CAD build for the part. Positions are in the model's coordinates, mm. Face numbers are marked on the shaded views. Coordinates: 2 decimals unless noted, no trailing zeros. Write each loop counter-clockwise with the first axis right and the second up, starting at its lowest first coordinate (ties: lowest second). Pieces come first, ordered by that corner, then holes. Notation, with made-up numbers: (-7.5, 54.5) - (32.5, 54.5) arc R20 ccw to (32.5, 63.5) - close; hole circle Ø8 at (18.5, -22). An arc over 180 degrees is marked (long way). One line per question, with ' | ' between items. Start each with the question number.
1. Two-plate mould, pull along Z, no slides. Class the marked faces 1, 2 and 3: +Z half, -Z half, draft (parallel to the pull), parting line (faces both ways), or undercut.
2. Band-saw the part on D-D, the plane x = -5. Write the cut outline in (y, z) (3 decimals), then the cut area to 3 significant figures.
3. Flat gauge pins, fed straight in: P1, Ø3, axis at x = -3.5, y = 19, coming from the -Z side; P2, Ø5.5, axis at y = 12.7, z = -19.05, coming from the +X side (1 decimal); P3, Ø6, axis at x = 0.5, y = 3, coming from the -Z side; P4, Ø4, axis at x = 4, z = -8, coming from the -Y side. Where does each tip first touch, or does it go through?
4. Band-saw the part on B-B, the plane z = -16.25. Write the cut outline in (x, y), then the cut area to 3 significant figures.
5. Probe line 1 (X direction, y = 8.5, z = -1); line 2 (Z direction, x = 3.75, y = 12.7) (3 decimals); line 3 (Z direction, x = -4.25, y = 23) (3 decimals). List the from-to ranges inside material, lowest first.
6. Band-saw the part on A-A, the plane y = 12.7. Write the cut outline in (x, z) (3 decimals).
7. Band-saw the part on C-C, the plane x = 5. Write the cut outline in (y, z) (3 decimals).
Autodesk Inventor part; units mm, degrees
ref_plane "YZ Plane" through (0, 0, 0) normal (1, 0, 0) x (0, 1, 0)
ref_plane "XZ Plane" through (0, 0, 0) normal (0, 1, 0) x (-1, 0, 0)
ref_plane "XY Plane" through (0, 0, 0) normal (0, 0, 1) x (1, 0, 0)
sketch "Sketch1" plane through (0, 0, 0) normal (1, 0, 0) x (0, 1, 0)
  line L0 (0, 0) -> (25.4, 0)
  line L1 (25.4, 0) -> (19.7868, -20.9489)
  line L2 (0, 0) -> (5.6132, -20.9489)
  line L3 (12.7, 0) -> (12.7, -162.0582)
  arc A0 (5.6132, -20.9489) -> (19.7868, -20.9489) centre (12.7, -19.05) ccw
  circle A1 centre (12.7, -19.05) radius 3.175
  dimension "d0" = 75
  dimension "d1" = 75
  dimension "d2" = 25.4
  dimension "d3" = 19.05
  dimension "d4" = 6.35
extrude "Extrusion1" add sketch "Sketch1" along normal blind 6.35 contours L0 L3 A1 A0 L2 | L0 L1 A0 L3 A1
sketch "Sketch2" plane through (0, 0, 0) normal (0, 0, 1) x (1, 0, 0)
  line L0 (6.35, 25.4) -> (-6.35, 25.4)
  line L1 (-6.35, 25.4) -> (-6.35, 0)
  line L2 (-6.35, 0) -> (6.35, 0)
  line L3 (6.35, 0) -> (6.35, 25.4)
  dimension "d7" = 12.7
extrude "Extrusion2" add sketch "Sketch2" along normal blind 3.175
equation "\"d1\" = d0"
properties part number "TabletMount-Base-Hinge"
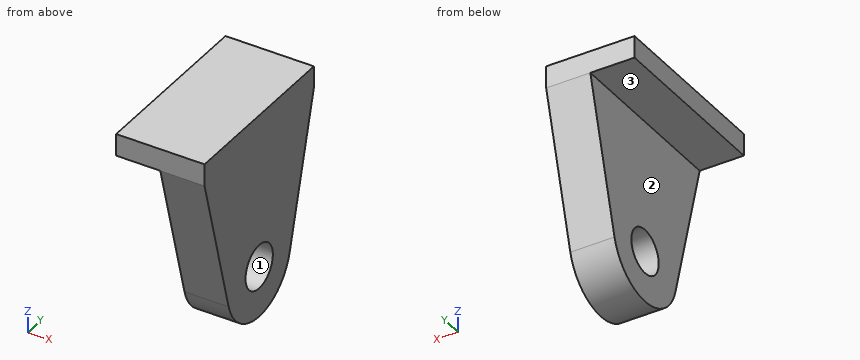
Filled in:
1) face 1: undercut | face 2: draft | face 3: -Z half
2) outline: (0, 0) - (25.4, 0) - (25.4, 3.175) - (0, 3.175) - close | area: 80.6 mm²
3) P1: stops at z = 0 | P2: passes through | P3: stops at z = -22.04 | P4: stops at y = 1.61
4) outline: (0, 4.35) - (6.35, 4.35) - (6.35, 11.2) - (0, 11.2) - close; (0, 14.2) - (6.35, 14.2) - (6.35, 21.05) - (0, 21.05) - close | area: 87.0 mm²
5) line 1: x = 0 to 6.35 | line 2: z = -26.387 to -22.225, -15.875 to 3.175 | line 3: z = 0 to 3.175
6) outline: (-6.35, 0) - (0, 0) - (0, -15.875) - (6.35, -15.875) - (6.35, 3.175) - (-6.35, 3.175) - close; (0, -26.387) - (6.35, -26.387) - (6.35, -22.225) - (0, -22.225) - close
7) outline: (0, 0) - (5.613, -20.949) arc R7.337 ccw to (19.787, -20.949) - (25.4, 0) - (25.4, 3.175) - (0, 3.175) - close; hole circle Ø6.35 at (12.7, -19.05)
